Answer from the drawing. Dimensions are ordinates in mm from the lowest x, y and z of the part. A direction names the side the tool comes from. Give positions to 0.01 mm unless a question says otherwise; leave off trailing zeros. Order: outer loops, then holes, each group sorted by start corner. A loop starts at its lowest first (then second) coordinate and runs counter-clockwise, first axis right, second up. Notation, with made-up numbers: (65.5, 42.5) -> (80.5, 42.5) arc R24 ccw to (80.5, 59.5) -> close; hole circle Ø2 at (3.5, 43). An arc over 180 degrees is marked (long way). Answer as a JSON object with one key per item and string values. Group by question number.
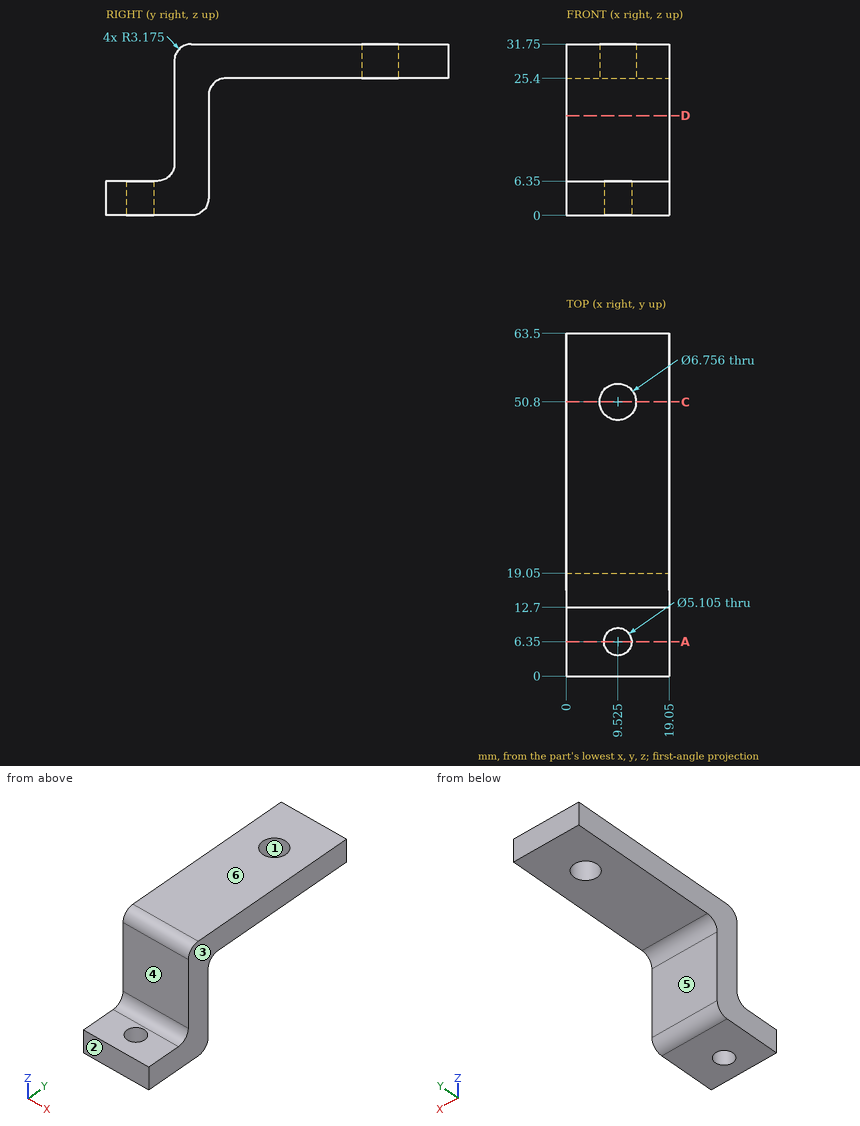
(1) For a pull along X with two mould halves and no side action, classify the marked faces 1, 2 and 3 as +X half, -X half, draft (parallel to the pull), parting line (faces both ways), or undercut.
(2) A cutting plane is placed at A-A (y = 6.35). Determine the outline of the cut face in (x, z).
(3) Find the intervals of material crossed by line 1 along X through (y, z) = (50.8, 27.25); line 2 along Z through (x, y) = (11.5, 33); line 3 along X through (y, z) = (6.35, 2), in increasing order. Write a range as [from, to].
(4) A cutting plane is placed at D-D (z = 18.5). Determine the outline of the cut face in (x, y), and give its area (3 significant figures).
(5) Which of the six approach directions +Z, -Z, +X, -X, +Y, -Y give full straight-line access (tool end or side, diameter ignored) to the marked faces 4, 5 and 6?
(6) Flat-ended cylindrical pins translate along their axes: pin 1 Ø8 at (x, z) = (4, 13) entering from -Y; pin 2 Ø8 at (x, y) = (5, 37) entering from -Z; pin 3 Ø7.5 at (x, y) = (12.5, 5) entering from +Z. Find the tip coordinate at first contact, or state that the pin passes through.
(7) A cutting plane is placed at C-C (y = 50.8). Determine the outline of the cut face in (x, z).
Check sheet entries:
{
 "1": {"face 1": "undercut", "face 2": "draft", "face 3": "+X half"},
 "2": {"outline": "(0, 0) -> (6.97, 0) -> (6.97, 6.35) -> (0, 6.35) -> close; (12.08, 0) -> (19.05, 0) -> (19.05, 6.35) -> (12.08, 6.35) -> close"},
 "3": {"line 1": "x = [0, 6.15], [12.9, 19.05]", "line 2": "z = [25.4, 31.75]", "line 3": "x = [0, 6.97], [12.08, 19.05]"},
 "4": {"outline": "(0, 12.7) -> (19.05, 12.7) -> (19.05, 19.05) -> (0, 19.05) -> close", "area": "121 mm2"},
 "5": {"face 4": "+Z, +X, -X, -Y", "face 5": "-Z, +X, -X, +Y", "face 6": "+Z, +X, -X, +Y, -Y"},
 "6": {"pin 1": "stops at y = 12.66", "pin 2": "stops at z = 25.4", "pin 3": "stops at z = 6.35"},
 "7": {"outline": "(0, 25.4) -> (6.15, 25.4) -> (6.15, 31.75) -> (0, 31.75) -> close; (12.9, 25.4) -> (19.05, 25.4) -> (19.05, 31.75) -> (12.9, 31.75) -> close"}
}
